Input: part model. Units: mm. Frame: model coordinates. A direction names the side the tool comes from. Round coordinates to 2 decimals unless told otherwise and drop trailing zeros. Loops run counter-clockwise (first coordinate to the right, second up) from the corner with the lowest first, then second, coordinate; pieces in that order, holes last. Notation, with made-up numbers: M 78,1 L 116,1 A16 cw 116,30 Z; hole C -3,-17 d9. An arc over 180 degrees is marked long. Return JSON: item names as keys, results as strings. Group by question number.
1) Section C-C (z = 0). Output: boundary loops of the cut face in (x, y), plus the area to 3 significant figures.
2) Access query for faces 5 (the face through (43, 17, -15)), 6 (the face through (27, 9, 17)), 7 (the face through (33.25, 21.48, 0.07)). Directions: +Z, -Z, +X, -X, +Y, -Y. A direction counts if a zero-diameter tool reaches every point of the face in a straight line with its end or side. Return the directions, or none.
3) Section D-D (y = 10.75). Output: boundary loops of the cut face in (x, z).
4) Section A-A (x = 12.5). Output: boundary loops of the cut face in (y, z).
5) Material intervals for line 1 (Z direction, x = 13.5, y = 6.5); line 2 (Y direction, x = 8.5, z = 9); line 3 (Y direction, x = 49, z = -16), sorted ascending. Write a range as from..to.
6) Contact query for flat-ended pins moving along their axis: P1, Ø8, axis at x = 7, z = 0, coming from the -Y side; P2, Ø0.9, axis at x = 43.5, z = 15, coming from the +Y side; P3, Ø0.9, axis at x = 16.5, y = 21.5, coming from the -Z side. Output: stop coordinate, or through.
7) Mould query, pull axis Z, two halves, no side actions, for faces 1 (the face through (27, 8, 14)), 2 (the face through (20, 23, -5)), 3 (the face through (19.72, 21.289, 15.196)), 4 (the face through (27, 9, -14)). Classes: +Z half, -Z half, draft (parallel to the pull), parting line (faces both ways), or undercut.
8) Section B-B (y = 13.5). Output: boundary loops of the cut face in (x, z), plus the area to 3 significant figures.
from build123d import *

# Parameters (mm, degrees)
BASE_FLANGE1_DEPTH       = 55
EXTRUDE1_START           = -23
EXTRUDE1_OUTLINE_W       = 15
EXTRUDE1_OUTLINE_H       = 36
EXTRUDE1_DEPTH           = 6
F_6_0_6_DIAMETER_HOLE1_D = 6
FILLET1_R                = 8
EXTRUDE2_DEPTH           = 61.942595941
FILLET2_R                = 8


# Read off the part's stored shape, not the designer's step: Extrude1
# Sheet-metal steps are written as plain solids
with BuildPart() as part:
    # Sketch1 → Base-Flange1 (new body)
    with BuildSketch(Plane(origin=(0, 0, 0), x_dir=(0, 0, -1), z_dir=(1, 0, 0))):
        with BuildLine():
            Line((-14, 0), (-14, 17))
            ThreePointArc((-14, 17), (-13.121320344, 19.121320344), (-11, 20))
            Line((-11, 20), (11, 20))
            ThreePointArc((11, 20), (13.121320344, 19.121320344), (14, 17))
            Line((14, 17), (14, 0))
            Line((14, 0), (17, 0))
            Line((17, 0), (17, 17))
            ThreePointArc((17, 17), (15.242640687, 21.242640687), (11, 23))
            Line((11, 23), (-11, 23))
            ThreePointArc((-11, 23), (-15.242640687, 21.242640687), (-17, 17))
            Line((-17, 17), (-17, 0))
            Line((-17, 0), (-14, 0))
        make_face()
    extrude(amount=BASE_FLANGE1_DEPTH)

    # Extrude1 outline → Extrude1 (cut)
    with BuildSketch(Plane.XZ.offset(EXTRUDE1_START)):
        with Locations((47.5, 0)):
            Rectangle(EXTRUDE1_OUTLINE_W, EXTRUDE1_OUTLINE_H)
    extrude(amount=EXTRUDE1_DEPTH, mode=Mode.SUBTRACT)

    # Ø6.0 (6) Diameter Hole1 (through all)
    with Locations(Plane.XY.offset(17)):
        with Locations((49, 8.5)):
            Hole(F_6_0_6_DIAMETER_HOLE1_D / 2)

    # Fillet1
    fillet1_edges = [part.edges().sort_by_distance(p)[0] for p in [
        (55, 0, 15.5),
        (55, 17, -15.5),
        (55, 17, 15.5),
        (55, 0, -15.5),
    ]]
    fillet(fillet1_edges, radius=FILLET1_R)

    # Sketch11 → Extrude2 (cut, through all)
    with BuildSketch(Plane.XZ.offset(-20)):
        with BuildLine():
            Line((10, 3.25), (30, 3.25))
            ThreePointArc((30, 3.25), (33.25, 0), (30, -3.25))
            Line((30, -3.25), (10, -3.25))
            ThreePointArc((10, -3.25), (6.75, 0), (10, 3.25))
        make_face()
    extrude(amount=-EXTRUDE2_DEPTH, mode=Mode.SUBTRACT)

    # Fillet2
    fillet2_edges = [part.edges().sort_by_distance(p)[0] for p in [
        (0, 0, 15.5),
        (0, 0, -15.5),
    ]]
    fillet(fillet2_edges, radius=FILLET2_R)


solid = part.part
Returned:
{
 "1": {"outline": "M 0,20 L 6.75,20 L 6.75,23 L 0,23 Z; M 33.25,20 L 40,20 L 40,23 L 33.25,23 Z", "area": "40.5 mm^2"},
 "2": {"face 5": "+Z, -Z, +X, +Y", "face 6": "+Z, +X, -X, +Y, -Y", "face 7": "+Y, -Y"},
 "3": {"outline": "M 0,-17 L 47.02,-17 L 47.02,-14 L 0,-14 Z; M 0,14 L 47.02,14 L 47.02,17 L 0,17 Z; M 50.98,-17 L 54.81,-17 L 54.81,-14 L 50.98,-14 Z; M 50.98,14 L 54.81,14 L 54.81,17 L 50.98,17 Z"},
 "4": {"outline": "M 0,-17 L 17,-17 A6 ccw 23,-11 L 23,-3.25 L 20,-3.25 L 20,-11 A3 cw 17,-14 L 0,-14 Z; M 0,14 L 17,14 A3 cw 20,11 L 20,3.25 L 23,3.25 L 23,11 A6 ccw 17,17 L 0,17 Z"},
 "5": {"line 1": "z = -17..-14, 14..17", "line 2": "y = 20..23", "line 3": "y = 0.25..5.5, 11.5..16.75"},
 "6": {"P1": "stops at y = 20", "P2": "stops at y = 17", "P3": "stops at z = -15.43"},
 "7": {"face 1": "undercut", "face 2": "draft", "face 3": "+Z half", "face 4": "undercut"},
 "8": {"outline": "M 0,-17 L 53.61,-17 L 53.61,-14 L 0,-14 Z; M 0,14 L 53.61,14 L 53.61,17 L 0,17 Z", "area": "322 mm^2"}
}
